CAD build for the part. Positions are in the model's coordinates, mm. Face numbers are marked on the shaded views. A direction names the side the tool comes from. Round coordinates to 2 decimals unless told otherwise and drop trailing zeros. Loops run counter-clockwise (first coordinate to the right, second up) from the corner with the lowest first, then second, coordinate; pieces in that order, holes last.
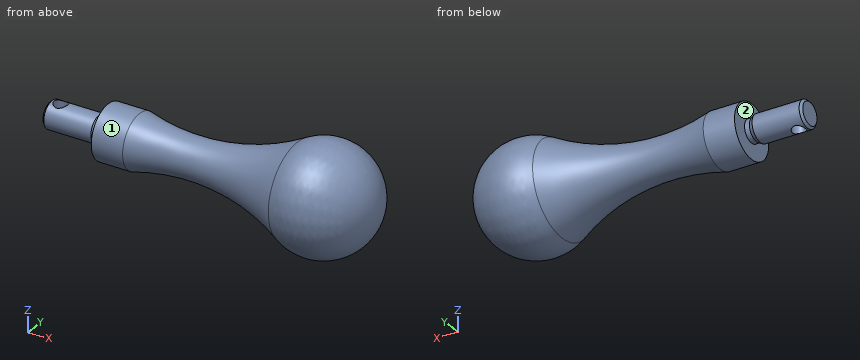
Autodesk Inventor part; units mm, degrees
ref_plane "Arbeitsebene1" through (-16.0421, -0.3839, 3) normal (0, 0, 1) x (1, 0, 0)
ref_plane "YZ Plane" through (0, 0, 0) normal (1, 0, 0) x (0, 1, 0)
ref_plane "XZ Plane" through (0, 0, 0) normal (0, 1, 0) x (-1, 0, 0)
sketch "Skizze1" plane through (0, 0, 0) normal (0, 0, 1) x (1, 0, 0)
  line L0 (51.4579, -0.3839) -> (-27.7559, -0.3839)
  arc A0 (51.4579, -0.3839) -> (33.7598, 9.9902) centre (39.5684, -0.3839) ccw
  arc A1 (-1.5421, 5.6161) -> (33.7598, 9.9902) centre (10.745, 51.0944) ccw
  line L1 (-1.5421, 5.6161) -> (-8.5421, 5.6161)
  line L2 (-8.5421, 5.6161) -> (-8.5421, -0.3839)
  line L3 (-8.5421, 2.1161) -> (-9.6248, 2.1161)
  line L4 (-9.6248, 2.1161) -> (-10.5421, 2.6161)
  line L5 (-10.5421, 2.6161) -> (-21.5421, 2.6161)
  line L6 (-21.5421, 2.6161) -> (-21.5421, -0.3839)
  dimension "d0" = 60
  dimension "d1" = 7
  dimension "d2" = 3
  dimension "d3" = 2.5
  dimension "d4" = 11
  dimension "d5" = 13
  dimension "d6" = 6
revolve "Drehung1" add sketch "Skizze1" angle 360 about axis through (51.4579, -0.3839, 0) along (-1, 0, 0)
chamfer "Fase1" distance 0.5 angle 45 1 edges at (-21.5421, -3.3839, 0)
thread "Gewinde1"
ref_plane "Arbeitsebene1" through (-16.0421, -0.3839, 3) normal (0, 0, 1) x (1, 0, 0)
sketch "Skizze2" plane through (-16.0421, -0.3839, 3) normal (0, 0, 1) x (1, 0, 0)
  line L0 (-5, 3) -> (-5, -3)
  line L1 (5.5, -3) -> (5.5, 3)
  line L2 (-5, 3) -> (-5, -3)
  line L3 (-5, 3) -> (5.5, 3)
  line L4 (-5, -3) -> (5.5, -3)
  line L5 (-5.5, -2.5) -> (-5.5, 2.5)
  point P0 (-3.1, 0)
  dimension "d14" = 3
  dimension "d15" = 2.4
hole "Bohrung1" at (-19.1421, -0.3839, 3) direction (0, 0, -1) diameter 3 end through all
properties part number "Glocke03"
Item 1: Flat gauge pins, fed straight in: P1, Ø8, axis at y = -6.5, z = -3.5, coming from the +X side; P2, Ø2, axis at x = 41.5, y = -7, coming from the -Z side; P3, Ø4, axis at y = 9, z = -8.5, coming from the +X side. Where does each tip first touch, or does it go through?
Answers follow:
P1: stops at x = 51.06
P2: stops at z = -10.33
P3: stops at x = 44.83
Item 2: Cut at A-A, the plane x = 0. Give the cut face in (y, z), plus the area to 3 significant figures.
Answers follow:
outline: circle Ø11.22 at (-0.38, 0)
area: 98.9 mm2
Item 3: 3-axis set-ups, long thin cutter, end or side, ignore diameter. For the marked faces 1 and 2: which of +Z, -Z, +X, -X, +Y, -Y reach the whole face in a straight line?
Answers follow:
face 1: -X
face 2: none
Item 4: Cut at B-B, the plane x = 7.5. Give the cut face in (y, z).
Answers follow:
outline: circle Ø8.96 at (-0.38, 0)
Item 5: Probe line 1 (X direction, y = 0, z = 0); line 2 (X direction, y = 3, z = -0.75); line 3 (Z direction, x = 17, y = -0.25). List the from-to ranges inside material, lowest first.
Answers follow:
line 1: x = -21.54 to -20.59, -17.69 to 51.45
line 2: x = -8.54 to 50.94
line 3: z = -4.78 to 4.78
